The listing builds one solid part. Answer for the finished solid, in the listing's coordinates (mm). Give positions to 0.01 mm unless a question says otherwise; leave off trailing zeros. Write each loop counter-clockwise with the first axis right and the second up, starting at its lowest first coordinate (ties: lowest second). Pieces come first, ordered by that corner, then holes. Notation, with made-up numbers: (-20.75, -15) - (-1.75, -15) arc R13 ccw to (-1.75, 7) - close; hole circle Ø11 at (-3.5, 23). An arc over 180 degrees is marked (long way). Answer as CSV lines item,"result". Start each with the question number.
(1) Straight lines are drawn through the part: probe 1 along Y at (x, z) = (16.5, 0.55); probe 2 along X at (y, z) = (2, 1.25); probe 3 along Y at (x, z) = (31.5, 1.5). For each, find the intervals that lie inside material, in ascending order.
(2) Find section C-C (y = 7.5). Write down the section's boundary in (x, z), then the cut area to 3 significant figures.
(3) Find section D-D (x = 31.5). Write down the section's boundary in (y, z).
(4) Find section A-A (z = 0.8). State how many separate pieces and enclosed holes the cut face has, then the cut area to 3 significant figures.
(5) Find section B-B (x = -20.5). Write down the section's boundary in (y, z), then the cut area to 3 significant figures.
from build123d import *

# Parameters (mm, degrees)
SKETCH_1_R      = 1.5
SKETCH_1_R_2    = 1.6
EXTRUDE_1_DEPTH = 2


with BuildPart() as part:
    # 草图1 → 凸台-拉伸1 (new body)
    with BuildSketch(Plane.XY):
        with BuildLine():
            Line((41.5, -24), (-41.5, -24))
            ThreePointArc((-41.5, -24), (-44.328427125, -22.828427125), (-45.5, -20))
            Line((-45.5, -20), (-45.5, 20))
            ThreePointArc((-45.5, 20), (-44.328427125, 22.828427125), (-41.5, 24))
            Line((-41.5, 24), (41.5, 24))
            ThreePointArc((41.5, 24), (44.328427125, 22.828427125), (45.5, 20))
            Line((45.5, 20), (45.5, -20))
            ThreePointArc((45.5, -20), (44.328427125, -22.828427125), (41.5, -24))
        make_face()
        with Locations((-31.5, 21)):
            Circle(SKETCH_1_R, mode=Mode.SUBTRACT)
        with Locations((31.5, 21)):
            Circle(SKETCH_1_R, mode=Mode.SUBTRACT)
        with Locations((31.5, -21)):
            Circle(SKETCH_1_R, mode=Mode.SUBTRACT)
        with Locations((-31.5, -21)):
            Circle(SKETCH_1_R, mode=Mode.SUBTRACT)
        with Locations((-41.5, 20)):
            Circle(SKETCH_1_R_2, mode=Mode.SUBTRACT)
        with Locations((-41.5, -20)):
            Circle(SKETCH_1_R_2, mode=Mode.SUBTRACT)
        with Locations((41.5, 20)):
            Circle(SKETCH_1_R_2, mode=Mode.SUBTRACT)
        with Locations((41.5, -20)):
            Circle(SKETCH_1_R_2, mode=Mode.SUBTRACT)
        with BuildLine():
            Line((29.5, -14), (-29.5, -14))
            ThreePointArc((-29.5, -14), (-35.156854249, -11.656854249), (-37.5, -6))
            Line((-37.5, -6), (-37.5, 6))
            ThreePointArc((-37.5, 6), (-35.156854249, 11.656854249), (-29.5, 14))
            Line((-29.5, 14), (29.5, 14))
            ThreePointArc((29.5, 14), (35.156854249, 11.656854249), (37.5, 6))
            Line((37.5, 6), (37.5, -6))
            ThreePointArc((37.5, -6), (35.156854249, -11.656854249), (29.5, -14))
        make_face(mode=Mode.SUBTRACT)
    extrude(amount=EXTRUDE_1_DEPTH)


solid = part.part
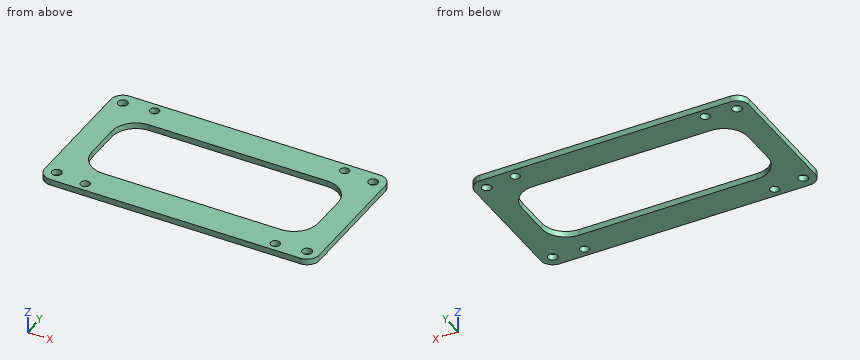
Result set:
1,probe 1,"-24 to -14, 14 to 24"
1,probe 2,"-45.5 to -37.5, 37.5 to 45.5"
1,probe 3,"-24 to -22.5, -19.5 to -13.75, 13.75 to 19.5, 22.5 to 24"
2,outline,"(-45.5, 0) - (-37.36, 0) - (-37.36, 2) - (-45.5, 2) - close; (37.36, 0) - (45.5, 0) - (45.5, 2) - (37.36, 2) - close"
2,area,"32.6 mm^2"
3,outline,"(-24, 0) - (-22.5, 0) - (-22.5, 2) - (-24, 2) - close; (-19.5, 0) - (-13.75, 0) - (-13.75, 2) - (-19.5, 2) - close; (13.75, 0) - (19.5, 0) - (19.5, 2) - (13.75, 2) - close; (22.5, 0) - (24, 0) - (24, 2) - (22.5, 2) - close"
4,separate pieces,"1"
4,enclosed holes,"9"
4,area,"2,250 mm^2"
5,outline,"(-24, 0) - (-14, 0) - (-14, 2) - (-24, 2) - close; (14, 0) - (24, 0) - (24, 2) - (14, 2) - close"
5,area,"40.0 mm^2"
